Part model, mm, in its own coordinate system. Round coordinates to 2 decimals unless told otherwise and drop trailing zeros. Write each loop counter-clockwise with the first axis right and the second up, starting at its lowest first coordinate (ties: lowest second). Pieces come first, ordered by that corner, then holes. Notation, with made-up numbers: (-28, 89.5) -> (1, 89.5) arc R18 cw to (1, 104.5) -> close; hole circle Ø1 at (84, 62.25). An arc over 180 degrees is marked (long way). Use CSV: the item, a comma, the result in double quotes. Start each with the question number.
Autodesk Inventor part; units mm, degrees
ref_plane "YZ Plane" through (0, 0, 0) normal (1, 0, 0) x (0, 1, 0)
ref_plane "XZ Plane" through (0, 0, 0) normal (0, 1, 0) x (-1, 0, 0)
ref_plane "XY Plane" through (0, 0, 0) normal (0, 0, 1) x (1, 0, 0)
sketch "Sketch1" plane through (0, 0, 0) normal (0, 1, 0) x (-1, 0, 0)
  line L0 (-2.4599, -13.6593) -> (-41.1266, -13.6593)
  arc A0 (-41.4599, -13.326) -> (-41.1266, -13.6593) centre (-41.1266, -13.326) ccw
  arc A1 (-2.4599, -13.6593) -> (-2.1266, -13.326) centre (-2.4599, -13.326) ccw
  line L1 (-2.1266, -13.326) -> (-2.1266, -10.9926)
  arc A2 (-2.1266, -10.9926) -> (-2.4599, -10.6593) centre (-2.4599, -10.9926) ccw
  line L2 (-2.4599, -10.6593) -> (-41.086, -5.9166)
  arc A3 (-41.086, -5.9166) -> (-41.4599, -6.2475) centre (-41.1266, -6.2475) ccw
  line L3 (-41.4599, -13.326) -> (-41.4599, -6.2475)
  point P0 (0, 0)
  dimension "d0" = 38.6667
  dimension "d1" = 0.6667
  dimension "d2" = 0.6667
  dimension "d4" = 0.6667
  dimension "d5" = 2.6667
  dimension "d6" = 7
  dimension "d7" = 0.6667
  dimension "d11" = 39.3333
extrude "Extrusion1" add sketch "Sketch1" along normal blind 6
properties part number "Wedge"
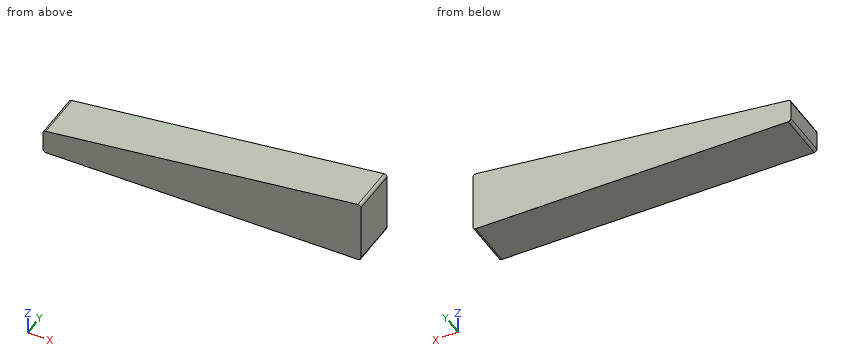
1. Band-saw the part on B-B (x = 17.5). List the corners of the cut face in (y, z), then the cut area to 3 significant figures.
2. Band-saw the part on C-C (z = -7). List the corners of the cut face in (x, y), then the cut area to 3 significant figures.
3. Flat gauge pin, fed straight in: pin 1 (2 mm diameter, centred on x = 30.5, y = 2.5, fed in from +Z). Where does the tip first touch, or does it go through?
4. Band-saw the part on A-A (y = 4.65). List the corners of the cut face in (x, z).
5. Drill centre lines: line 1 along Z through (x, y) = (15, 1.85); line 2 along Z through (x, y) = (4, 4.85). Where is each one in solid material? Low to high. Write a range as [from, to].
Answers below:
1,outline,"(0, -13.66) -> (6, -13.66) -> (6, -8.81) -> (0, -8.81) -> close"
1,area,"29.1 mm^2"
2,outline,"(32.26, 0) -> (41.46, 0) -> (41.46, 6) -> (32.26, 6) -> close"
2,area,"55.2 mm^2"
3,pin 1,"stops at z = -7.09"
4,outline,"(2.13, -13.33) arc R0.33 ccw to (2.46, -13.66) -> (41.13, -13.66) arc R0.33 ccw to (41.46, -13.33) -> (41.46, -6.25) arc R0.33 ccw to (41.09, -5.92) -> (2.46, -10.66) arc R0.33 ccw to (2.13, -10.99) -> close"
5,line 1,"z = [-13.66, -9.12]"
5,line 2,"z = [-13.66, -10.47]"
